```python
from build123d import *

# Parameters (mm, degrees)
BOSS_EXTRUDE1_DEPTH = 25.4


with BuildPart() as part:
    # Sketch1 → Boss-Extrude1 (new body)
    with BuildSketch(Plane(origin=(0, 0, 0), x_dir=(1, 0, 0), z_dir=(0, 1, 0))):
        with BuildLine():
            ThreePointArc((-11.307534998, 15.331084511), (-0.657073574, 19.03866472), (10.223658013, 16.074181685))
            Line((10.223658013, 16.074181685), (47.730081944, -7.781020346))
            ThreePointArc((47.730081944, -7.781020346), (56.527791269, -22.811130875), (49.427965792, -38.713847313))
            Line((49.427965792, -38.713847313), (36.32387238, -49.227658983))
            ThreePointArc((36.32387238, -49.227658983), (61.722416996, -31.519775069), (51.137967948, -2.422959784))
            Line((51.137967948, -2.422959784), (13.631544017, 21.432242246))
            ThreePointArc((13.631544017, 21.432242246), (-0.876098099, 25.384886293), (-15.07671333, 20.441446014))
            Line((-15.07671333, 20.441446014), (-47.420289399, -3.413756016))
            ThreePointArc((-47.420289399, -3.413756016), (-57.694182826, -22.271934185), (-49.846542995, -42.261889641))
            Line((-49.846542995, -42.261889641), (-51.320154567, -25.526120494))
            ThreePointArc((-51.320154567, -25.526120494), (-49.708739726, -16.022348708), (-43.651111067, -8.52411752))
            Line((-43.651111067, -8.52411752), (-11.307534998, 15.331084511))
        make_face()
    extrude(amount=BOSS_EXTRUDE1_DEPTH)


solid = part.part
```
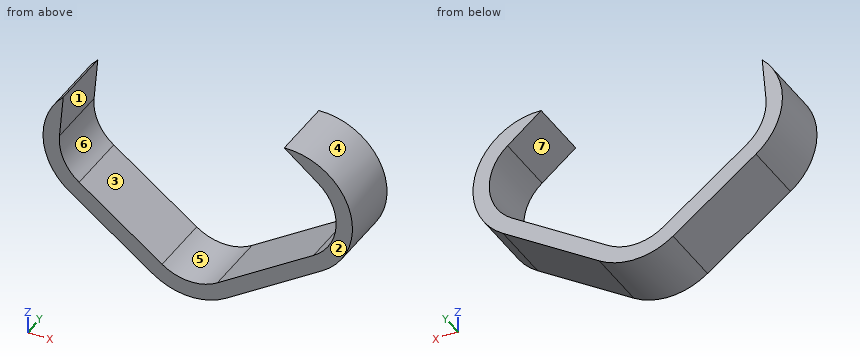
Check sheet for the modelled part. Datum: model origin and axes. Units: mm. Face numbers are marked on the shaded views. A direction names the side the tool comes from. Give positions to 0.01 mm unless a question says otherwise; leave off trailing zeros. Write each loop counter-clockwise with the first axis right and the second up, starting at its lowest first coordinate (ties: lowest second). Pieces come first, ordered by that corner, then holes. Notation, with made-up numbers: (38.25, 20) - (91.25, 20) arc R34 cw to (91.25, 50) - close; hole circle Ø9 at (69.25, 53). An arc over 180 degrees is marked (long way). Answer as a JSON object with one key per item and string values. Group by question number.
1) Sectioned sample at C-C (y = 18). Record the cut outline in (x, z).
2) Release check for a two-part mould opening along Z. For the marked faces 4, 5, 6 and 7 record: pulls with the +Z half, pulls with the -Z half, needs draft (parallel to the pull), parting line crosses it, or undercut.
3) Sectioned sample at B-B (x = 41.5). Record the cut outline in (y, z), then the cut area to 3 significant figures.
4) Thickness scan on probe 1 along X at (y, z) = (7, 9.5); probe 2 along X at (y, z) = (22.75, -16.5); probe 3 along Z at (x, y) = (-1, 14.5). Record the ranges inside material, lowest first. Write a range as from..to.
5) Depth check by flat-ended pin: P1, Ø1, axis at x = 25, z = -16, coming from the +Y side; P2, Ø1, axis at x = 16.5, y = 13.5, coming from the +Z side; P3, Ø1.5, axis at x = -40, y = 15.5, coming from the -Z side; P4, Ø1, axis at y = 16, z = 3.5, coming from the -X side. Enter the tip coordinate at first touch or a pass-through.
6) Sectioned sample at D-D (x = -41). Record the cut outline in (y, z).
7) Access from +Z, -Z, +X, -X, +Y, -Y to the whole of each face (thin tool, end or side, straight path). Record for the marked faces 1, 2 and 3.
8) Sectioned sample at A-A (z = 36.5). Record the cut outline in (x, y).
Geometry results:
{
 "1": {"outline": "(-51.32, 25.53) - (-49.85, 42.26) arc R25.4 ccw to (-47.42, 3.41) - (-15.08, -20.44) arc R25.4 ccw to (13.63, -21.43) - (51.14, 2.42) arc R25.4 ccw to (36.32, 49.23) - (49.43, 38.71) arc R19.05 cw to (47.73, 7.78) - (10.22, -16.07) arc R19.05 cw to (-11.31, -15.33) - (-43.65, 8.52) arc R19.05 cw to start"},
 "2": {"face 4": "parting line crosses it", "face 5": "pulls with the +Z half", "face 6": "undercut", "face 7": "undercut"},
 "3": {"outline": "(0, -3.71) - (25.4, -3.71) - (25.4, 3.82) - (0, 3.82) - close; (0, 45.07) - (25.4, 45.07) - (25.4, 48.94) - (0, 48.94) - close", "area": "289 mm^2"},
 "4": {"probe 1": "x = -53.3..-44.87, 50.03..58.46", "probe 2": "x = -20.42..-9.52, 9.52..21.39", "probe 3": "z = -25.38..-19.02"},
 "5": {"P1": "passes through", "P2": "stops at z = -11.76", "P3": "stops at z = -2.61", "P4": "stops at x = -48.18"},
 "6": {"outline": "(0, -1.32) - (25.4, -1.32) - (25.4, 6.57) - (0, 6.57) - close"},
 "7": {"face 1": "+Y, -Y", "face 2": "+Z, -Z, +X, -X, -Y", "face 3": "+Z, +Y, -Y"},
 "8": {"outline": "(-54.37, 0) - (-50.35, 0) - (-50.35, 25.4) - (-54.37, 25.4) - close; (51.75, 0) - (59.54, 0) - (59.54, 25.4) - (51.75, 25.4) - close"}
}
